The model under review builds one solid part; all positions refer to its coordinate system, in mm. Face numbers are marked on the shaded views. A direction names the side the tool comes from. Round coordinates to 2 decimals unless told otherwise and drop trailing zeros. Order: outer loops, then holes, each group sorted by start corner. A loop starts at its lowest first (then second) coordinate and runs counter-clockwise, first axis right, second up. Notation, with made-up numbers: M -28,-14.5 L 20,-14.5 A13 ccw 20,6.5 Z; hole C 86.5,-4 d10. An arc over 180 degrees is marked long. Answer as a JSON object with one key per item and string values. Group by question number.
1) Consider section C-C, the plane z = 1.25. Write out the cut boundary in (x, y), then the cut area to 3 significant figures.
2) Insertion check: pin 1 Ø4 at (x, z) = (-3, 1) entering from +Y; pin 2 Ø3.5 at (x, z) = (-5, 6) entering from -Y. Each pin has a flat end and moves straight along its axis. Give the tip position at first contact, or say it passes through.
3) For the marked faces 4, 5 and 6, list the 3-axis set-ups (+Z, -Z, +X, -X, +Y, -Y) from which the entire face can be reached by the end or side of a thin tool; tool diameter is ignored.
4) Consider section A-A, the plane x = 0. Write out the cut boundary in (y, z), then the cut area to 3 significant figures.
5) Consider section D-D, the plane x = -2.25. Write out the cut boundary in (y, z), then the cut area to 3 significant figures.
6) The part is to be moulded in two halves that separate along X. For the marked faces 1, 2 and 3, say which applies: +X half, -X half, draft (parallel to the pull), parting line (faces both ways), or undercut.
7) Consider section B-B, the plane z = 3.5. Write out the cut boundary in (x, y), then the cut area to 3 significant figures.
8) To check wall thickness, follow line 1 (X direction, y = 0, z = 2.25); line 2 (Z direction, x = -6.5, y = 0.75); line 3 (Y direction, x = -4.75, z = 5.75). State the ranges of each line that lie inside material, in increasing order.
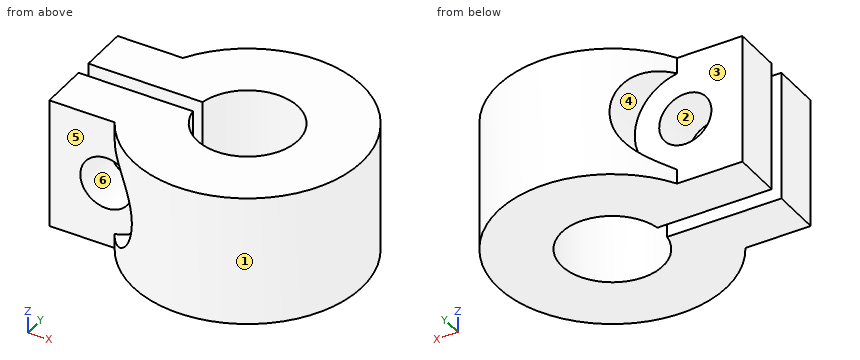
```python
from build123d import *

# Parameters (mm, degrees)
BOSS_EXTRUDE1_DEPTH = 8
SKETCH2_R           = 1.6
CUT_EXTRUDE1_DEPTH  = 17.598115032
SKETCH3_R           = 3.1
CUT_EXTRUDE2_DEPTH  = 17.598115143
SKETCH4_R           = 3.1
CUT_EXTRUDE3_DEPTH  = 17.598115143


with BuildPart() as part:
    # Sketch1 → Boss-Extrude1 (new body)
    with BuildSketch(Plane.XY):
        with BuildLine():
            Line((-6.062177826, 3.5), (-10.062177826, 3.5))
            Line((-10.062177826, 3.5), (-10.062177826, 0.5))
            Line((-10.062177826, 0.5), (-3.059411708, 0.5))
            ThreePointArc((-3.059411708, 0.5), (3.1, 0), (-3.059411708, -0.5))
            Line((-3.059411708, -0.5), (-10.062177826, -0.5))
            Line((-10.062177826, -0.5), (-10.062177826, -3.5))
            Line((-10.062177826, -3.5), (-6.062177826, -3.5))
            ThreePointArc((-6.062177826, -3.5), (7, 0), (-6.062177826, 3.5))
        make_face()
    extrude(amount=BOSS_EXTRUDE1_DEPTH)

    # Sketch2 → Cut-Extrude1 (cut, through all)
    with BuildSketch(Plane(origin=(0, 3.5, 0), x_dir=(1, 0, 0), z_dir=(0, 1, 0))):
        with Locations(Location((-6.562177826, -3.951427487, 0), (0, 0, 90))):
            Circle(SKETCH2_R)
    extrude(amount=-CUT_EXTRUDE1_DEPTH, mode=Mode.SUBTRACT)

    # Sketch3 → Cut-Extrude2 (cut, through all)
    with BuildSketch(Plane(origin=(0, 3.5, 0), x_dir=(1, 0, 0), z_dir=(0, 1, 0))):
        with Locations((-6.562177826, -3.951427487)):
            Circle(SKETCH3_R)
    extrude(amount=CUT_EXTRUDE2_DEPTH, mode=Mode.SUBTRACT)

    # Sketch4 → Cut-Extrude3 (cut, through all)
    with BuildSketch(Plane.XZ.offset(3.5)):
        with Locations((-6.562177826, 3.951427487)):
            Circle(SKETCH4_R)
    extrude(amount=CUT_EXTRUDE3_DEPTH, mode=Mode.SUBTRACT)


solid = part.part
```
Results list:
{
 "1": {"outline": "M -10.06,-3.5 L -5.04,-3.5 L -5.04,-4.86 A7 ccw long -5.04,4.86 L -5.04,3.5 L -10.06,3.5 L -10.06,0.5 L -3.06,0.5 A3.1 cw long -3.06,-0.5 L -10.06,-0.5 Z", "area": "139 mm^2"},
 "2": {"pin 1": "y = 6.93", "pin 2": "y = -6.2"},
 "3": {"face 4": "-X, +Y", "face 5": "-X, -Y", "face 6": "+Y, -Y"},
 "4": {"outline": "M -7,0 L -3.1,0 L -3.1,8 L -7,8 Z; M 3.1,0 L 7,0 L 7,8 L 3.1,8 Z", "area": "62.4 mm^2"},
 "5": {"outline": "M -6.63,0 L -2.13,0 L -2.13,8 L -6.63,8 Z; M 2.13,0 L 6.63,0 L 6.63,8 L 2.13,8 Z", "area": "71.9 mm^2"},
 "6": {"face 1": "parting line", "face 2": "undercut", "face 3": "draft"},
 "7": {"outline": "M -10.06,-3.5 L -8.1,-3.5 L -8.1,-0.5 L -10.06,-0.5 Z; M -10.06,0.5 L -8.1,0.5 L -8.1,3.5 L -10.06,3.5 Z; M -5.03,-3.5 L -3.5,-3.5 L -3.5,-6.06 A7 ccw long -3.5,6.06 L -3.5,3.5 L -5.03,3.5 L -5.03,0.5 L -3.06,0.5 A3.1 cw long -3.06,-0.5 L -5.03,-0.5 Z", "area": "114 mm^2"},
 "8": {"line 1": "3.1 to 7", "line 2": "0 to 2.35, 5.55 to 8", "line 3": "-3.5 to -0.5, 0.5 to 3.5"}
}
